Autodesk Inventor part; units mm, degrees
ref_plane "YZ Plane" through (0, 0, 0) normal (1, 0, 0) x (0, 1, 0)
ref_plane "XZ Plane" through (0, 0, 0) normal (0, 1, 0) x (-1, 0, 0)
ref_plane "XY Plane" through (0, 0, 0) normal (0, 0, 1) x (1, 0, 0)
sketch "Esquisse1" plane through (0, 0, 0) normal (0, 1, 0) x (-1, 0, 0)
  line L0 (-17.8264, 13.8129) -> (-17.8264, 6.3115)
  line L1 (20.1692, 13.8129) -> (-17.8264, 13.8129)
  line L2 (20.1692, 6.3115) -> (20.1692, 13.8129)
  line L3 (20.1692, 6.3115) -> (20.1692, 5.0615)
  arc A0 (19.9192, 4.8115) -> (20.1692, 5.0615) centre (19.9192, 5.0615) ccw
  line L4 (16.2667, 4.8115) -> (19.9192, 4.8115)
  arc A1 (16.2667, 4.8115) -> (16.0167, 4.5615) centre (16.2667, 4.5615) ccw
  line L5 (16.0167, -1.9385) -> (16.0167, 4.5615)
  arc A2 (16.0167, -1.9385) -> (16.2667, -2.1885) centre (16.2667, -1.9385) ccw
  line L6 (18.6692, -2.1885) -> (16.2667, -2.1885)
  arc A3 (18.6692, -2.1885) -> (18.9192, -1.9385) centre (18.6692, -1.9385) ccw
  line L7 (18.9192, 2.8115) -> (18.9192, -1.9385)
  arc A4 (18.9192, 3.8115) -> (18.9192, 2.8115) centre (18.9192, 3.3115) ccw
  line L8 (19.9192, 3.8115) -> (18.9192, 3.8115)
  arc A5 (20.1692, 3.5615) -> (19.9192, 3.8115) centre (19.9192, 3.5615) ccw
  line L9 (20.1692, 3.5615) -> (20.1692, -3.6892)
  line L10 (20.1692, -11.1878) -> (20.1692, -3.6892)
  line L11 (20.1692, -11.1878) -> (-17.8264, -11.1878)
  line L12 (-17.8264, -3.6892) -> (-17.8264, -11.1878)
  line L13 (-17.8264, 3.5615) -> (-17.8264, -3.6892)
  arc A6 (-17.5764, 3.8115) -> (-17.8264, 3.5615) centre (-17.5764, 3.5615) ccw
  line L14 (-16.5764, 3.8115) -> (-17.5764, 3.8115)
  arc A7 (-16.5764, 2.8115) -> (-16.5764, 3.8115) centre (-16.5764, 3.3115) ccw
  line L15 (-16.5764, -1.9385) -> (-16.5764, 2.8115)
  arc A8 (-16.5764, -1.9385) -> (-16.3264, -2.1885) centre (-16.3264, -1.9385) ccw
  line L16 (-13.9239, -2.1885) -> (-16.3264, -2.1885)
  arc A9 (-13.9239, -2.1885) -> (-13.6739, -1.9385) centre (-13.9239, -1.9385) ccw
  line L17 (-13.6739, 4.5615) -> (-13.6739, -1.9385)
  arc A10 (-13.6739, 4.5615) -> (-13.9239, 4.8115) centre (-13.9239, 4.5615) ccw
  line L18 (-17.5764, 4.8115) -> (-13.9239, 4.8115)
  arc A11 (-17.8264, 5.0615) -> (-17.5764, 4.8115) centre (-17.5764, 5.0615) ccw
  line L19 (-17.8264, 6.3115) -> (-17.8264, 5.0615)
  circle A12 centre (-14.8286, -6.6881) radius 1
  circle A13 centre (-14.8286, 9.3119) radius 1
  circle A14 centre (17.1714, 9.3119) radius 1
  circle A15 centre (17.1714, -6.6881) radius 1
  circle A16 centre (-6.8286, -6.6881) radius 1
  circle A17 centre (-6.8286, 9.3119) radius 1
  circle A18 centre (9.1714, 9.3119) radius 1
  circle A19 centre (9.1714, -6.6881) radius 1
  circle A20 centre (-6.8286, 1.3119) radius 1
  circle A21 centre (1.1714, 9.3119) radius 1
  circle A22 centre (9.1714, 1.3119) radius 1
  circle A23 centre (1.1714, -6.6881) radius 1
  line L20 (6.1717, 4.2695) -> (6.1717, -1.6458)
  line L21 (3.8644, 4.2695) -> (6.1717, 4.2695)
  arc A24 (3.8644, 4.2695) -> (-1.5216, 4.2695) centre (1.1714, 1.3119) ccw
  line L22 (-3.8289, 4.2695) -> (-1.5216, 4.2695)
  line L23 (-3.8289, -1.6458) -> (-3.8289, 4.2695)
  line L24 (-1.5216, -1.6458) -> (-3.8289, -1.6458)
  arc A25 (-1.5216, -1.6458) -> (3.8644, -1.6458) centre (1.1714, 1.3119) ccw
  line L25 (6.1717, -1.6458) -> (3.8644, -1.6458)
  line L26 (-17.8264, 13.8129) -> (20.1692, 13.8129)
  line L27 (20.1692, 13.8129) -> (20.1692, -11.1878)
  line L28 (20.1692, -11.1878) -> (-17.8264, -11.1878)
  line L29 (-17.8264, -11.1878) -> (-17.8264, 13.8129)
  circle A26 centre (-6.8286, -6.6881) radius 1
  circle A27 centre (-6.8286, 1.3119) radius 1
  circle A28 centre (-6.8286, 9.3119) radius 1
  circle A29 centre (1.1714, 9.3119) radius 1
  circle A30 centre (1.1714, -6.6881) radius 1
  circle A31 centre (9.1714, -6.6881) radius 1
  circle A32 centre (9.1714, 1.3119) radius 1
  circle A33 centre (9.1714, 9.3119) radius 1
extrude "Extrusion1" add sketch "Esquisse1" along normal blind 10 contours L1 L2 L3 A0 L4 A1 L5 A2 L6 A3 L7 A4 L8 A5 L9 L10 L11 L12 L13 A6 L14 A7 L15 A8 L16 A9 L17 A10 L18 A11 L19 L0 | A11 L18 A10 L17 A9 L16 A8 L15 A7 L14 A6 L29 | L27 A5 L8 A4 L7 A3 L6 A2 L5 A1 L4 A0 | A12 | A13 | A14 | A15 | L20 L25 A25 L24 L23 L22 A24 L21
sketch "Esquisse2" plane through (0, 0, 0) normal (0, -1, 0) x (1, 0, 0)
  circle A0 centre (-56.1714, 1.3122) radius 30
  line L0 (-61.1714, 36.3122) -> (-40.1692, 36.3122)
  line L1 (-20.1692, 16.3122) -> (-20.1692, -13.6878)
  line L2 (-40.1692, -33.6878) -> (-61.1714, -33.6878)
  line L3 (-91.1714, -3.6878) -> (-91.1714, 6.3122)
  arc A1 (-61.1714, 36.3122) -> (-91.1714, 6.3122) centre (-61.1714, 6.3122) ccw
  arc A2 (-91.1714, -3.6878) -> (-61.1714, -33.6878) centre (-61.1714, -3.6878) ccw
  line L4 (-20.1692, -11.1878) -> (-20.1692, 13.8129)
  arc A3 (-20.1692, 16.3122) -> (-40.1692, 36.3122) centre (-40.1692, 16.3122) ccw
  arc A4 (-40.1692, -33.6878) -> (-20.1692, -13.6878) centre (-40.1692, -13.6878) ccw
  point P0 (0, 0)
  dimension "d4" = 35
  dimension "d5" = 35
  dimension "d6" = 35
  dimension "d7" = 30
  dimension "d8" = 30
  dimension "d9" = 0
  dimension "d10" = 20
  dimension "d11" = 20
extrude "Extrusion2" add sketch "Esquisse2" against normal blind 10
sketch "Esquisse3" plane through (-61.1714, 0, 36.3122) normal (0, 0, 1) x (1, 0, 0)
  line L0 (35, 92.5) -> (35, -82.5)
  circle A0 centre (5, 5) radius 1.5
  line L1 (0, 10) -> (21.0022, 10)
  point P0 (61.1714, 0)
  dimension "d14" = 30
  dimension "d15" = 3
  dimension "d16" = 5
extrude "Extrusion3" cut sketch "Esquisse3" against normal through all
sketch "Esquisse4" plane through (-91.1714, 0, -3.6878) normal (-1, 0, 0) x (0, 0, 1)
  line L0 (35, 92.5) -> (35, -82.5)
  circle A0 centre (5, 5) radius 1.5
  line L1 (0, 0) -> (10, 0)
  point P0 (3.6878, 0)
  dimension "d19" = 3
  dimension "d20" = 30
  dimension "d21" = 5
extrude "Extrusion4" cut sketch "Esquisse4" against normal up to next
sketch "Esquisse5" plane through (0, 0, 0) normal (0, -1, 0) x (1, 0, 0)
  circle A0 centre (-56.1714, 1.3122) radius 30.5
  circle A1 centre (-56.1714, 1.3122) radius 30
  point P0 (0, 0)
  dimension "d25" = 61
  dimension "d26" = 0
  dimension "d27" = 0
extrude "Extrusion5" cut sketch "Esquisse5" against normal through all
properties part number "rotation-recuperation"
The model under review builds one solid part; all positions refer to its coordinate system, in mm. A direction names the side the tool comes from. Give positions to 0.01 mm unless a question says otherwise; leave off trailing zeros. Write each loop counter-clockwise with the first axis right and the second up, starting at its lowest first coordinate (ties: lowest second). Pieces come first, ordered by that corner, then holes.
1. Add section D-D, the plane x = 4.5. Write out the cut boundary in (y, z), plus the area to 3 significant figures.
2. Add section B-B, the plane x = -46. Write out the cut boundary in (y, z), plus the area to 3 significant figures.
3. Draft analysis for pull direction Z (two halves, no side actions). For faces 5 (the cylindrical face through (-27.08, 4.93, 10.47)), 6 (the cylindrical face through (-25.872, 4.93, 30.298)), 7 (the cylindrical face through (-57.362, 4.087, -31.388)), 8 (the cylindrical face through (-10.095, 4.93, 1.695)), state which applies: +Z half, -Z half, draft (parallel to the pull), parting line (faces both ways), or undercut.
4. For P1, Ø1, axis at x = -11.5, y = 6.5, coming from the -Z side; P2, Ø3, axis at x = -71, y = 1.5, coming from the -Z side; P3, Ø1.5, axis at y = 8.5, z = -10, coming from the -X side, all flat-tipped, find the tip position at first contact; note any pin that passes through.
5. Tool access review of faces 1 (the flat face through (-1, 5, -11.188)), 2 (the cylindrical face through (-88.93, 4.09, 0.12)), 3 (the flat face through (-91.171, 3.8, 0.1)), 4 (the flat face through (-1, 5, 13.813)): name each direction out of +Z, -Z, +X, -X, +Y, -Y from which nothing blocks a thin tool from reaching the whole face with its end or side.
6. Add section C-C, the plane y = 5. Count the separate pieces of the cut face and the enclosed holes in it, plus the area to 3 significant figures.
7. Add section A-A, the plane z = -2. Write out the cut boundary in (x, y).
8. Wall thickness on L1, parallel to Z at x = -1.5, y = 4.25; L2, parallel to Z at x = -3, y = 2.75; L3, parallel to Z at x = -60, y = 1.75: over which ranges is each line inside the solid? List them lowest first.
Worked answers:
1. outline: (0, -11.19) - (10, -11.19) - (10, 13.81) - (0, 13.81) - close
1. area: 250 mm2
2. outline: (0, -33.69) - (10, -33.69) - (10, -27.44) - (0, -27.44) - close; (0, 30.07) - (10, 30.07) - (10, 36.31) - (0, 36.31) - close
2. area: 125 mm2
3. face 5: undercut
3. face 6: +Z half
3. face 7: draft
3. face 8: undercut
4. P1: stops at z = -11.19
4. P2: stops at z = -32.51
4. P3: stops at x = -90.65
5. face 1: -Z, +X, +Y, -Y
5. face 2: -X
5. face 3: +Z, -Z, -X, +Y, -Y
5. face 4: +Z, +X, +Y, -Y
6. separate pieces: 3
6. enclosed holes: 8
6. area: 2,370 mm2
7. outline: (-91.17, 0) - (-86.49, 0) - (-86.49, 10) - (-91.17, 10) - close; (-25.85, 0) - (17.83, 0) - (17.83, 10) - (-25.85, 10) - close
8. L1: z = -11.19 to -7.63, -5.74 to 8.37, 10.26 to 13.81
8. L2: z = -11.19 to 13.81
8. L3: z = -33.69 to -28.95, 31.57 to 36.31
